Autodesk Inventor part; units mm, degrees
ref_plane "YZ Plane" through (0, 0, 0) normal (1, 0, 0) x (0, 1, 0)
ref_plane "XZ Plane" through (0, 0, 0) normal (0, 1, 0) x (-1, 0, 0)
ref_plane "XY Plane" through (0, 0, 0) normal (0, 0, 1) x (1, 0, 0)
sketch "Эскиз1" plane through (0, 0, 0) normal (0, 0, 1) x (1, 0, 0)
  circle A0 centre (0, 2.5) radius 1.1
  circle A1 centre (55, 2.5) radius 1.1
  circle A2 centre (0, 57.5) radius 1.1
  circle A3 centre (55, 57.5) radius 1.1
  line L0 (15.5, 60) -> (0, 60)
  line L1 (-2.5, 57.5) -> (-2.5, 2.5)
  line L2 (55, 60) -> (39.5, 60)
  line L3 (57.5, 2.5) -> (57.5, 57.5)
  line L4 (-2.5, 2.5) -> (-2.5, 0)
  line L5 (0, 60) -> (-2.5, 60)
  line L6 (-2.5, 60) -> (-2.5, 57.5)
  line L7 (39.5, 60) -> (15.5, 60)
  line L8 (57.5, 2.5) -> (57.5, 0)
  line L9 (57.5, 0) -> (-2.5, 0)
  line L10 (57.5, 57.5) -> (57.5, 60)
  line L11 (57.5, 60) -> (55, 60)
  line L12 (-7.5, 63.5411) -> (62.5, 63.5411)
  line L13 (62.5, 63.5411) -> (62.5, -3.5411)
  line L14 (62.5, -3.5411) -> (-7.5, -3.5411)
  line L15 (-7.5, -3.5411) -> (-7.5, 63.5411)
  line L16 (-7.5, 63.5411) -> (62.5, -3.5411) construction
  line L17 (62.5, 63.5411) -> (-7.5, -3.5411) construction
  point P0 (0, 0)
  point P1 (27.5, 30)
  dimension "d0" = 70
extrude "Выдавливание1" add sketch "Эскиз1" along normal blind 5 contours A0 | A1 | A2 | A3 | L7 L2 L11 L10 L3 L8 L9 L4 L1 L6 L5 L0 | L12 L13 L14 L15
sketch "Эскиз2" plane through (0, 0, 0) normal (0, 0, -1) x (-1, 0, 0)
  line L0 (7.5, 63.5411) -> (7.5, -3.5411)
  line L1 (-62.5, -3.5411) -> (-62.5, 63.5411)
  line L2 (-62.5, 63.5411) -> (7.5, 63.5411)
  line L3 (7.5, -3.5411) -> (-62.5, -3.5411)
  line L4 (12.5, 70) -> (-67.5, 70)
  line L5 (-67.5, 70) -> (-67.5, -10)
  line L6 (-67.5, -10) -> (12.5, -10)
  line L7 (12.5, -10) -> (12.5, 70)
  line L8 (12.5, 70) -> (-67.5, -10) construction
  line L9 (-67.5, 70) -> (12.5, -10) construction
  point P0 (0, 0)
  point P1 (-27.5, 30)
  dimension "d3" = 80
  dimension "d4" = 80
extrude "Выдавливание2" add sketch "Эскиз2" against normal blind 30
sketch "Эскиз3" plane through (0, 0, 5) normal (0, 0, 1) x (1, 0, 0)
  circle A0 centre (55, 2.5) radius 1.75
  circle A1 centre (55, 57.5) radius 1.75
  circle A2 centre (0, 57.5) radius 1.75
  circle A3 centre (0, 2.5) radius 1.75
  point P0 (0, 0)
  dimension "d7" = 3.5
  dimension "d8" = 3.5
  dimension "d9" = 3.5
  dimension "d10" = 3.5
extrude "Выдавливание3" cut sketch "Эскиз3" against normal blind 4
fillet "Сопряжение1" radius 5 4 edges at (67.5, -10, 15) (67.5, 70, 15) (-12.5, -10, 15) (-12.5, 70, 15)
sketch "Эскиз5" plane through (0, 0, 30) normal (0, 0, 1) x (1, 0, 0)
  circle A0 centre (0, 57.5) radius 1.75
  line L0 (0, 57.5) -> (0, 63.5411)
  line L1 (62.5, 63.5411) -> (-7.5, 63.5411)
  line L2 (-7.5, 70) -> (62.5, 70)
  line L3 (0, 70) -> (0, 63.5411)
  circle A1 centre (55, 57.5) radius 1.75
  line L4 (55, 57.5) -> (55, 63.5411)
  line L5 (55, 63.5411) -> (55, 70)
  circle A2 centre (55, 66.7706) radius 1.75
  circle A3 centre (0, 66.7706) radius 1.75
  circle A4 centre (55, 2.5) radius 1.75
  line L6 (55, 2.5) -> (55, -3.5411)
  line L7 (62.5, -3.5411) -> (-7.5, -3.5411)
  line L8 (55, -3.5411) -> (55, -10)
  line L9 (62.5, -10) -> (-7.5, -10)
  circle A5 centre (0, 2.5) radius 1.75
  line L10 (0, 2.5) -> (0, -3.5411)
  line L11 (0, -3.5411) -> (0, -10)
  circle A6 centre (55, -6.7706) radius 1.75
  circle A7 centre (0, -6.7706) radius 1.75
  point P0 (0, 0)
  dimension "d14" = 3.5
  dimension "d15" = 3.5
  dimension "d16" = 3.5
  dimension "d17" = 3.5
extrude "Выдавливание4" cut sketch "Эскиз5" against normal blind 4 contours A3 L3 | L3 A3 | A2 L5 | L5 A2 | A6 L8 | L8 A6 | A7 L11 | L11 A7
sketch "Эскиз6" plane through (0, 0, 30) normal (0, 0, 1) x (1, 0, 0)
  line L0 (62.5, 70) -> (-7.5, 70)
  line L1 (-12.5, 65) -> (-12.5, -5)
  arc A0 (-7.5, 70) -> (-12.5, 65) centre (-7.5, 65) ccw
  arc A1 (67.5, 65) -> (62.5, 70) centre (62.5, 65) ccw
  line L2 (67.5, -5) -> (67.5, 65)
  arc A2 (62.5, -10) -> (67.5, -5) centre (62.5, -5) ccw
  line L3 (-7.5, -10) -> (62.5, -10)
  arc A3 (-12.5, -5) -> (-7.5, -10) centre (-7.5, -5) ccw
  circle A4 centre (0, 66.7706) radius 1.75
  circle A5 centre (55, 66.7706) radius 1.75
  circle A6 centre (55, -6.7706) radius 1.75
  circle A7 centre (0, -6.7706) radius 1.75
  line L4 (62.5, -3.5411) -> (-7.5, -3.5411)
  line L5 (-7.5, -3.5411) -> (-7.5, 63.5411)
  line L6 (-7.5, 63.5411) -> (62.5, 63.5411)
  line L7 (62.5, 63.5411) -> (62.5, -3.5411)
  point P0 (0, 0)
sketch "Эскиз7" plane through (67.5, -5, 0) normal (1, 0, 0) x (0, 0, -1)
  line L0 (-30, -5) -> (0, -5)
  line L1 (-30, 0) -> (-30, 70)
  line L2 (0, 75) -> (-30, 75)
  line L3 (0, 70) -> (0, 0)
  line L4 (-30, 35) -> (0, 35)
  line L5 (-12.99, 13.983) -> (-12.99, 13.543)
  line L6 (-12.55, 13.543) -> (-12.55, 13.983)
  line L7 (-12.99, 13.763) -> (-12.55, 13.763)
  line L8 (-13.44, 12.493) -> (-12.1, 12.493)
  line L9 (-16.77, 9) -> (-8.77, 9)
  line L10 (-8.77, 9) -> (-8.77, 61)
  line L11 (-8.77, 61) -> (-16.77, 61)
  line L12 (-16.77, 61) -> (-16.77, 9)
  line L13 (-12.77, 13.763) -> (-12.77, 10.2135)
  point P0 (0, 5)
  dimension "d20" = 26
  dimension "d21" = 26
  dimension "d22" = 8
  dimension "d23" = 4
extrude "Выдавливание5" cut sketch "Эскиз7" against normal through all
sketch "Эскиз8" plane through (-7.5, -10, 0) normal (0, -1, 0) x (1, 0, 0)
  line L0 (32, 26.125) -> (38, 26.125)
  line L1 (34.72, 23.225) -> (32.7, 23.225)
  line L2 (30.9, 24.9) -> (30.9, 25.1)
  line L3 (39.1, 25.1) -> (39.1, 24.9)
  line L4 (30.9, 25.1) -> (30.9, 26.125)
  line L5 (30.9, 26.125) -> (39.1, 26.125)
  line L6 (39.1, 26.125) -> (39.1, 23.225)
  line L7 (39.1, 23.225) -> (30.9, 23.225)
  line L8 (30.9, 23.225) -> (30.9, 25.1)
  line L9 (42.5, 20.675) -> (27.5, 20.675)
  line L10 (27.5, 20.675) -> (27.5, 28.675)
  line L11 (27.5, 28.675) -> (42.5, 28.675)
  line L12 (42.5, 28.675) -> (42.5, 20.675)
  line L13 (42.5, 20.675) -> (27.5, 28.675) construction
  line L14 (27.5, 20.675) -> (42.5, 28.675) construction
  line L15 (42.5, 21.175) -> (27.5, 21.175)
  line L16 (27.5, 21.175) -> (27.5, 28.175)
  line L17 (27.5, 28.175) -> (42.5, 28.175)
  line L18 (42.5, 28.175) -> (42.5, 21.175)
  line L19 (42.5, 21.175) -> (27.5, 28.175) construction
  line L20 (27.5, 21.175) -> (42.5, 28.175) construction
  point P0 (7.5, 0)
  point P1 (35, 24.675)
  dimension "d26" = 15
  dimension "d27" = 8
  dimension "d28" = 15
  dimension "d29" = 7
extrude "Выдавливание6" cut sketch "Эскиз8" against normal blind 10 contours L0 L5 L6 L3 L7 L1 L8 L2 L4 | L15 L10 L17 L12
properties part number "Case_Base"
The model under review builds one solid part; all positions refer to its coordinate system, in mm. A direction names the side the tool comes from. Round coordinates to 2 decimals unless told otherwise and drop trailing zeros. Write each loop counter-clockwise with the first axis right and the second up, starting at its lowest first coordinate (ties: lowest second). Pieces come first, ordered by that corner, then holes.
(1) Machinability: for faces 5 (the flat face through (35, -7, 25)), 6 (the flat face through (65, 30, 16.77)), 7 (the flat face through (0, 67, 26)), 8 (the flat face through (28, -5, 30)), which of the approach directions +Z, -Z, +X, -X, +Y, -Y give a long, thin tool a straight path to every point of the face, cutting with its end or side? Answer none if there is none.
(2) We need section C-C on y = 2.5. Give the boundary of the cut face in (x, z).
(3) Insertion check: pin 1 (4 mm diameter, centred on x = -10.5, z = 14, fed in from +Y); pin 2 (1 mm diameter, centred on x = 54.5, y = 66, fed in from +Z); pin 3 (4 mm diameter, centred on x = 54.5, y = 3, fed in from +Z). Each pin has a flat end and moves straight along its axis. Give the tip position at first contact, or say it passes through.
(4) We need section A-A on z = 13.25. Give the boundary of the cut face in (x, y), and give its area (3 significant figures).
(5) Wall thickness on L1, parallel to Y at x = 0, z = 27.4; L2, parallel to Y at x = 55, z = 3.65; L3, parallel to X at y = 45, z = 8: over which ranges is each line inside the solid? List them lowest first.
(6) We need section D-D on z = 24.75. Give the boundary of the cut face in (x, y).
(7) We need section B-B on y = 42.5. Give the boundary of the cut face in (x, z), and give its area (3 significant figures).
(8) Mouldability with a two-part tool opening along Y and no side actions: class faces 1 (the cylindrical face through (-11.07, -8.5, 15.21)), 2 (the flat face through (-12.5, 30, 18)), 3 (the cylindrical face through (-11, 68.57, 15.21)), 4 (the flat face through (55, 67, 26)) as +Y half, -Y half, draft (parallel to the pull), parting line (faces both ways), or undercut.
Findings below:
1. face 5: -Y
1. face 6: +X, -X
1. face 7: +Z
1. face 8: +Z, +X, -X, +Y, -Y
2. outline: (-12.5, 0) - (67.5, 0) - (67.5, 30) - (62.5, 30) - (62.5, 5) - (56.75, 5) - (56.75, 1) - (53.25, 1) - (53.25, 5) - (1.75, 5) - (1.75, 1) - (-1.75, 1) - (-1.75, 5) - (-7.5, 5) - (-7.5, 30) - (-12.5, 30) - close
3. pin 1: stops at y = 69.9
3. pin 2: stops at z = 26
3. pin 3: stops at z = 5
4. outline: (-12.5, -5) arc R5 ccw to (-7.5, -10) - (62.5, -10) arc R5 ccw to (67.5, -5) - (67.5, 4) - (62.5, 4) - (62.5, -3.54) - (-7.5, -3.54) - (-7.5, 4) - (-12.5, 4) - close; (-12.5, 56) - (-7.5, 56) - (-7.5, 63.54) - (62.5, 63.54) - (62.5, 56) - (67.5, 56) - (67.5, 65) arc R5 ccw to (62.5, 70) - (-7.5, 70) arc R5 ccw to (-12.5, 65) - close
4. area: 1,160 mm2
5. L1: y = -10 to -8.52, -5.02 to -3.54, 63.54 to 65.02, 68.52 to 70
5. L2: y = -10 to 0.75, 4.25 to 55.75, 59.25 to 70
5. L3: x = -12.5 to -7.5, 62.5 to 67.5
6. outline: (-12.5, -5) arc R5 ccw to (-7.5, -10) - (20, -10) - (20, -3.54) - (-7.5, -3.54) - (-7.5, 63.54) - (62.5, 63.54) - (62.5, -3.54) - (35, -3.54) - (35, -10) - (62.5, -10) arc R5 ccw to (67.5, -5) - (67.5, 65) arc R5 ccw to (62.5, 70) - (-7.5, 70) arc R5 ccw to (-12.5, 65) - close
7. outline: (-12.5, 0) - (67.5, 0) - (67.5, 8.77) - (62.5, 8.77) - (62.5, 5) - (-7.5, 5) - (-7.5, 8.77) - (-12.5, 8.77) - close; (-12.5, 16.77) - (-7.5, 16.77) - (-7.5, 30) - (-12.5, 30) - close; (62.5, 16.77) - (67.5, 16.77) - (67.5, 30) - (62.5, 30) - close
7. area: 570 mm2
8. face 1: -Y half
8. face 2: draft
8. face 3: +Y half
8. face 4: undercut
